```python
from build123d import *

# Parameters (mm, degrees)
SKETCH1_W           = 150
SKETCH1_H           = 90
BOSS_EXTRUDE1_DEPTH = 50
BOSS_EXTRUDE2_START = -100
SKETCH2_W           = 200
SKETCH2_H           = 200
BOSS_EXTRUDE2_DEPTH = 200
SKETCH3_W           = 150
SKETCH3_H           = 150
CUT_EXTRUDE1_DEPTH  = 200
SKETCH4_W           = 15
SKETCH4_H           = 15
SKETCH4_H_2         = 12.5
SKETCH4_W_2         = 35
BOSS_EXTRUDE3_DEPTH = 200
SKETCH6_W           = 15
SKETCH6_H           = 15
BOSS_EXTRUDE4_DEPTH = 200
SKETCH5_R           = 15
BOSS_EXTRUDE5_DEPTH = 95
SKETCH7_W           = 150
SKETCH7_H           = 55
CUT_EXTRUDE2_DEPTH  = 200


with BuildPart() as part:
    # Sketch1 → Boss-Extrude1 (new body)
    with BuildSketch(Plane(origin=(0, 0, 0), x_dir=(1, 0, 0), z_dir=(0, 1, 0))):
        Rectangle(SKETCH1_W, SKETCH1_H)
    extrude(amount=BOSS_EXTRUDE1_DEPTH)

    # Sketch2 → Boss-Extrude2 (add)
    with BuildSketch(Plane.XY.offset(BOSS_EXTRUDE2_START)):
        with Locations((0, 150)):
            Rectangle(SKETCH2_W, SKETCH2_H)
    extrude(amount=BOSS_EXTRUDE2_DEPTH)

    # Sketch3 → Cut-Extrude1 (cut)
    with BuildSketch(Plane.XY.offset(100)):
        with Locations((0, 150)):
            Rectangle(SKETCH3_W, SKETCH3_H)
    extrude(amount=-CUT_EXTRUDE1_DEPTH, mode=Mode.SUBTRACT)

    # Sketch4 → Boss-Extrude3 (add)
    with BuildSketch(Plane.XY.offset(100)):
        with Locations((0, 205)):
            Rectangle(SKETCH4_W, SKETCH4_H)
        with Locations((0, 218.75)):
            Rectangle(SKETCH4_W, SKETCH4_H_2)
        with Locations((-25, 205)):
            Rectangle(SKETCH4_W_2, SKETCH4_H)
        with Locations((25, 205)):
            Rectangle(SKETCH4_W_2, SKETCH4_H)
        with Locations((0, 191.25)):
            Rectangle(SKETCH4_W, SKETCH4_H_2)
        with Locations((0, 108.75)):
            Rectangle(SKETCH4_W, SKETCH4_H_2)
        with Locations((0, 95)):
            Rectangle(SKETCH4_W, SKETCH4_H)
        with Locations((0, 81.25)):
            Rectangle(SKETCH4_W, SKETCH4_H_2)
        with Locations((-25, 95)):
            Rectangle(SKETCH4_W_2, SKETCH4_H)
        with Locations((25, 95)):
            Rectangle(SKETCH4_W_2, SKETCH4_H)
    extrude(amount=-BOSS_EXTRUDE3_DEPTH)

    # Sketch6 → Boss-Extrude4 (add)
    with BuildSketch(Plane.XY.offset(100)):
        with Locations((0, 185)):
            Rectangle(SKETCH6_W, SKETCH6_H)
        with Locations((0, 115)):
            Rectangle(SKETCH6_W, SKETCH6_H)
    extrude(amount=-BOSS_EXTRUDE4_DEPTH)

    # Sketch5 → Boss-Extrude5 (add)
    with BuildSketch(Plane.XZ.offset(-197.5)):
        with Locations(Location((35, 75, 0), (0, 0, 60))):
            Circle(SKETCH5_R)
        with Locations(Location((35, 25, 0), (0, 0, 60))):
            Circle(SKETCH5_R)
        with Locations(Location((35, -25, 0), (0, 0, 60))):
            Circle(SKETCH5_R)
        with Locations(Location((35, -75, 0), (0, 0, 60))):
            Circle(SKETCH5_R)
        with Locations(Location((-35, 75, 0), (0, 0, 120))):
            Circle(SKETCH5_R)
        with Locations(Location((-35, 25, 0), (0, 0, 120))):
            Circle(SKETCH5_R)
        with Locations(Location((-35, -25, 0), (0, 0, 120))):
            Circle(SKETCH5_R)
        with Locations(Location((-35, -75, 0), (0, 0, 120))):
            Circle(SKETCH5_R)
    extrude(amount=BOSS_EXTRUDE5_DEPTH)

    # Sketch7 → Cut-Extrude2 (cut)
    with BuildSketch(Plane.XY.offset(100)):
        with Locations((0, 150)):
            Rectangle(SKETCH7_W, SKETCH7_H)
    extrude(amount=-CUT_EXTRUDE2_DEPTH, mode=Mode.SUBTRACT)


solid = part.part
```
Can you work these out from the model? Positions are in its coordinate system, mm. A direction names the side the tool comes from. Round coordinates to 2 decimals unless told otherwise and drop trailing zeros. Order: outer loops, then holes, each group sorted by start corner. A loop starts at its lowest first (then second) coordinate and runs counter-clockwise, first axis right, second up. Notation, with made-up numbers: (-9, -31.5) -> (10, -31.5) arc R8 cw to (10, -18.5) -> close; hole circle Ø6 at (86, 28). An arc over 180 degrees is marked (long way). Return JSON: item names as keys, results as strings. Group by question number.
1. If we section it at A-A, the plane y = 79: Write out the boundary of the cut face in (x, z).
2. Which directions (+Z, -Z, +X, -X, +Y, -Y) give clear straight access to the entire face, cutting with the end or side of a thin tool? Please do faces 3 (the face through (-26.94, 187.64, -62.35)), 4 (the face through (0, 177.5, 1)).
3. I need wall thicknesses on line 1 (Y direction, x = -31, z = 51); line 2 (Y direction, x = 9, z = -31.5); line 3 (X direction, y = 218.5, z = 4.5). Which ranges of each line are inside material? Lowest first, please. Write a range as [from, to].
4. If we section it at C-C, the plane y = 130: Write out the boundary of the cut face in (x, z).
5. Will this pin go through, and if not, where does the flat tip stop? pin 1 (6 mm diameter, centred on x = -46.5, z = -77, fed in from -Y).
6. If we section it at D-D, the plane x = 35: Count the separate pieces of the cut face and the enclosed holes in it, then the cut area to 3 significant figures.
7. We'd pull the mould along X, two halves only. Please class faces 1 (the face through (7.5, 81, 1)), 2 (the face through (-1, 107, -100)): released by +X, released by -X, zero draft, split by the parting line, or undercut.
Output values:
{
 "1": {"outline": "(-100, -100) -> (-75, -100) -> (-75, 100) -> (-100, 100) -> close; (-7.5, -100) -> (7.5, -100) -> (7.5, 100) -> (-7.5, 100) -> close; (75, -100) -> (100, -100) -> (100, 100) -> (75, 100) -> close"},
 "2": {"face 3": "none", "face 4": "+Z, -Z"},
 "3": {"line 1": "[50, 75], [87.5, 102.5], [197.5, 212.5], [225, 250]", "line 2": "[0, 75], [87.5, 102.5], [197.5, 212.5], [225, 250]", "line 3": "[-100, -75], [-7.5, 7.5], [75, 100]"},
 "4": {"outline": "(-100, -100) -> (-75, -100) -> (-75, 100) -> (-100, 100) -> close; (75, -100) -> (100, -100) -> (100, 100) -> (75, 100) -> close"},
 "5": {"pin 1": "y = 50"},
 "6": {"separate pieces": "4", "enclosed holes": "0", "area": "25,300 mm²"},
 "7": {"face 1": "undercut", "face 2": "zero draft"}
}
